Can you work these out from the drawing? Everything is in mm from the part's minimum corner. A direction names the side the tool comes from. Coordinates: 2 decimals unless noted, no trailing zeros. Order: outer loops, then holes, each group sorted by start corner. A loop starts at its lowest first (then second) coordinate and runs counter-clockwise, first axis right, second up. Notation, with made-up numbers: (75.5, -6.75) - (95.5, -6.75) arc R34 ccw to (95.5, 28.25) - close; hole circle Ø6 at (-19.5, 23). An arc over 180 degrees is marked (long way). Answer as CSV lines item,"result". Start each with the question number.
Item 1: Imagine slicing it at B-B on z = 47. List the corners of the cut face in (x, y) for me (1 decimal), and give its area (3 significant figures).
Item 2: Imagine slicing it at C-C on y = 223. List the corners of the cut face in (x, z) for me (1 decimal), and give its area (3 significant figures).
Item 3: On a 3-axis mill with a long thin cutter (end or side, diameter ignored), from which of +Z, -Z, +X, -X, +Y, -Y can I reach the whole of each face in a straight line? I mean the marked faces 1, 2, 3 and 4. Say none if no direction works.
Item 4: I need wall thicknesses on line 1 (Y direction, x = 6.5, z = 47.5); line 2 (X direction, y = 151, z = 37); line 3 (Y direction, x = 54.5, z = 33). Which ranges of each line are inside material? Lowest first, please.
Item 5: Imagine slicing it at D-D on z = 36. List the corners of the cut face in (x, y) for me (1 decimal).
Item 6: Imagine slicing it at A-A on x = 51.5. List the corners of the cut face in (y, z) for me, and give its area (3 significant figures).
Item 7: I'm going to push flat-ended pins straight in: pin 1 (6 mm diameter, centred on x = 11.5, z = 38, fed in from +Y); pin 2 (5.5 mm diameter, centred on y = 196, z = 37, fed in from +X); pin 3 (9.5 mm diameter, centred on x = 42.5, y = 229.5, fed in from -Z); pin 4 (4 mm diameter, centred on x = 62, y = 96, fed in from -Z). Where does each tip first touch, or does it pass through?
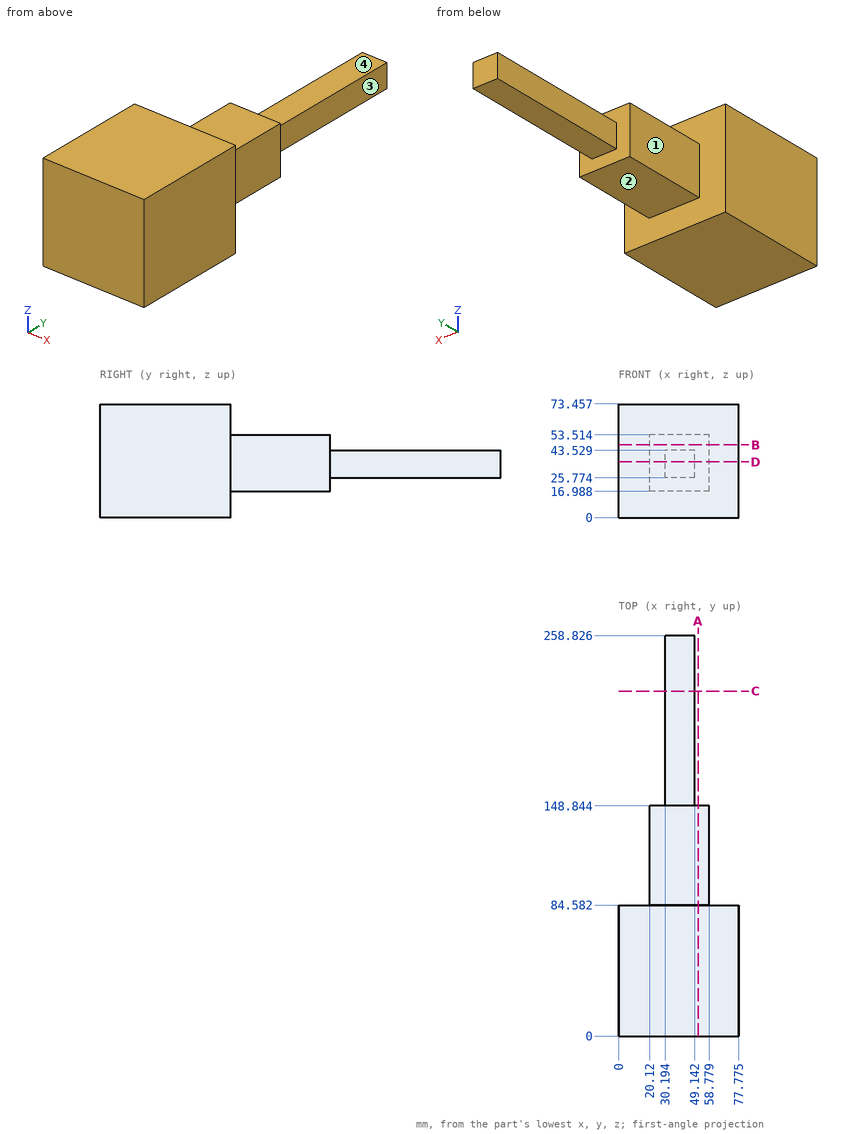
Responses:
1,outline,"(0, 0) - (77.8, 0) - (77.8, 84.6) - (58.8, 84.6) - (58.8, 148.8) - (20.1, 148.8) - (20.1, 84.6) - (0, 84.6) - close"
1,area,"9,060 mm^2"
2,outline,"(30.2, 25.8) - (49.1, 25.8) - (49.1, 43.5) - (30.2, 43.5) - close"
2,area,"336 mm^2"
3,face 1,"+Z, -Z, -X, +Y"
3,face 2,"-Z, +X, -X, +Y"
3,face 3,"+Z, -Z, +X, +Y"
3,face 4,"+Z, +X, -X, +Y"
4,line 1,"y = 0 to 84.58"
4,line 2,"x = 30.19 to 49.14"
4,line 3,"y = 0 to 148.84"
5,outline,"(0, 0) - (77.8, 0) - (77.8, 84.6) - (58.8, 84.6) - (58.8, 148.8) - (49.1, 148.8) - (49.1, 258.8) - (30.2, 258.8) - (30.2, 148.8) - (20.1, 148.8) - (20.1, 84.6) - (0, 84.6) - close"
6,outline,"(0, 0) - (84.58, 0) - (84.58, 16.99) - (148.84, 16.99) - (148.84, 53.51) - (84.58, 53.51) - (84.58, 73.46) - (0, 73.46) - close"
6,area,"8,560 mm^2"
7,pin 1,"stops at y = 84.58"
7,pin 2,"stops at x = 49.14"
7,pin 3,"stops at z = 25.77"
7,pin 4,"passes through"
